from build123d import *

# Parameters (mm, degrees)
SKETCH_1_R      = 25.25
EXTRUDE_1_DEPTH = 1.6
EXTRUDE_2_DEPTH = 1.6


with BuildPart() as part:
    # 草图1 → 凸台-拉伸1 (new body)
    with BuildSketch(Plane(origin=(0, 0, 0), x_dir=(1, 0, 0), z_dir=(0, 1, 0))):
        with Locations(Location((0, 0, 0), (0, 0, 270))):
            Circle(SKETCH_1_R)
    extrude(amount=EXTRUDE_1_DEPTH)

    # 草图2 → 凸台-拉伸2 (add)
    with BuildSketch(Plane(origin=(0, 1.6, 0), x_dir=(1, 0, 0), z_dir=(0, 1, 0))):
        with BuildLine():
            Line((-20.506096654, 24.748737342), (0, 4.242640687))
            Line((0, 4.242640687), (20.506096654, 24.748737342))
            ThreePointArc((20.506096654, 24.748737342), (24.748737342, 24.748737342), (24.748737342, 20.506096654))
            Line((24.748737342, 20.506096654), (4.242640687, 0))
            Line((4.242640687, 0), (24.748737342, -20.506096654))
            ThreePointArc((24.748737342, -20.506096654), (24.748737342, -24.748737342), (20.506096654, -24.748737342))
            Line((20.506096654, -24.748737342), (0, -4.242640687))
            Line((0, -4.242640687), (-20.506096654, -24.748737342))
            ThreePointArc((-20.506096654, -24.748737342), (-24.748737342, -24.748737342), (-24.748737342, -20.506096654))
            Line((-24.748737342, -20.506096654), (-4.242640687, 0))
            Line((-4.242640687, 0), (-24.748737342, 20.506096654))
            ThreePointArc((-24.748737342, 20.506096654), (-24.748737342, 24.748737342), (-20.506096654, 24.748737342))
        make_face()
        with BuildLine():
            Line((-21.531401487, 23.723432509), (-17.854446225, 20.046477247))
            ThreePointArc((-17.854446225, 20.046477247), (-17.854446225, 17.854446225), (-20.046477247, 17.854446225))
            Line((-20.046477247, 17.854446225), (-23.723432509, 21.531401487))
            ThreePointArc((-23.723432509, 21.531401487), (-23.723432509, 23.723432509), (-21.531401487, 23.723432509))
        make_face(mode=Mode.SUBTRACT)
        with BuildLine():
            Line((23.723432509, 21.531401487), (20.046477247, 17.854446225))
            ThreePointArc((20.046477247, 17.854446225), (17.854446225, 17.854446225), (17.854446225, 20.046477247))
            Line((17.854446225, 20.046477247), (21.531401487, 23.723432509))
            ThreePointArc((21.531401487, 23.723432509), (23.723432509, 23.723432509), (23.723432509, 21.531401487))
        make_face(mode=Mode.SUBTRACT)
        with BuildLine():
            Line((21.531401487, -23.723432509), (17.854446225, -20.046477247))
            ThreePointArc((17.854446225, -20.046477247), (17.854446225, -17.854446225), (20.046477247, -17.854446225))
            Line((20.046477247, -17.854446225), (23.723432509, -21.531401487))
            ThreePointArc((23.723432509, -21.531401487), (23.723432509, -23.723432509), (21.531401487, -23.723432509))
        make_face(mode=Mode.SUBTRACT)
        with BuildLine():
            Line((-23.723432509, -21.531401487), (-20.046477247, -17.854446225))
            ThreePointArc((-20.046477247, -17.854446225), (-17.854446225, -17.854446225), (-17.854446225, -20.046477247))
            Line((-17.854446225, -20.046477247), (-21.531401487, -23.723432509))
            ThreePointArc((-21.531401487, -23.723432509), (-23.723432509, -23.723432509), (-23.723432509, -21.531401487))
        make_face(mode=Mode.SUBTRACT)
    extrude(amount=-EXTRUDE_2_DEPTH)


solid = part.part
CAD build for the part. Positions are in the model's coordinates, mm. A direction names the side the tool comes from. Round coordinates to 2 decimals unless told otherwise and drop trailing zeros. Order: outer loops, then holes, each group sorted by start corner. A loop starts at its lowest first (then second) coordinate and runs counter-clockwise, first axis right, second up. Notation, with made-up numbers: (17.5, 37.25) -> (47.5, 37.25) arc R20 ccw to (47.5, 66.25) -> close; hole circle Ø4 at (-1, 15). An arc over 180 degrees is marked (long way). Write item = value, one per line. Start each with the question number.
(1) Probe line 1 (Z direction, x = 18, y = 1.3); line 2 (X direction, y = 0.25, z = -22); line 3 (Z direction, x = -21, y = 0.6). List the from-to ranges inside material, lowest first. Write a range as [from, to].
(2) Cut at D-D, the plane x = -6. List the corners of the cut face in (y, z), then the cut area to 3 significant figures.
(3) Pull direction Z, two halves, no side cores. Call faces 5 (the flat face through (21.91, 0.81, -19.72)), 6 (the cylindrical face through (0.24, 0.79, -25.25)), 7 (the flat face through (0, 1.6, 0)): released by +Z, released by -Z, zero draft, split by the parting line, or undercut.
(4) Cut at A-A, the plane y = 1. State how many separate pieces and enclosed holes the cut face has, then the cut area to 3 significant figures.
(5) Which spindle directions (+Z, -Z, +X, -X, +Y, -Y) get a long thin tool onto all of the face, cutting with end or side? Do faces 1 (the flat face through (18.02, 0.81, -22.26)), 2 (the flat face through (-19.67, 0.81, 21.86)), 3 (the flat face through (22.33, 0.81, -18.09)), 4 (the flat face through (-22.26, 0.81, -18.02)). Say none if no direction does.
(6) Cut at C-C, the plane z = -12.5. List the corners of the cut face in (x, y).
(7) Cut at B-B, the plane x = -19. List the corners of the cut face in (y, z), then the cut area to 3 significant figures.
Model answer:
q1.line_1 = [-22.24, -20.19], [-17.73, 17.73], [20.19, 22.24]
q1.line_2 = [-25.56, -24.04], [-19.81, -17.76], [-12.39, 12.39], [17.76, 19.81], [24.04, 25.56]
q1.line_3 = [-25.15, -23.19], [-18.81, -16.76], [-14.02, 14.02], [16.76, 18.81], [23.19, 25.15]
q2.outline = (0, -24.53) -> (1.6, -24.53) -> (1.6, 24.53) -> (0, 24.53) -> close
q2.area = 78.5 mm2
q3.face_5 = undercut
q3.face_6 = released by -Z
q3.face_7 = zero draft
q4.separate_pieces = 1
q4.enclosed_holes = 4
q4.area = 2,130 mm2
q5.face_1 = -Z, +Y, -Y
q5.face_2 = +Y, -Y
q5.face_3 = +X, +Y, -Y
q5.face_4 = -X, +Y, -Y
q6.outline = (-21.94, 0) -> (21.94, 0) -> (21.94, 1.6) -> (-21.94, 1.6) -> close
q7.outline = (0, -23.24) -> (1.6, -23.24) -> (1.6, -21.19) -> (0, -21.19) -> close; (0, -17.4) -> (1.6, -17.4) -> (1.6, 17.4) -> (0, 17.4) -> close; (0, 21.19) -> (1.6, 21.19) -> (1.6, 23.24) -> (0, 23.24) -> close
q7.area = 62.2 mm2
